Input: part model. Units: mm. Frame: model coordinates. Face numbers are marked on the shaded views. Give positions to 0.01 mm unless a question says otherwise; leave off trailing zeros. Loops run counter-clockwise (first coordinate to the right, second up) from the corner with the lowest first, then second, coordinate; pieces in that order, holes last. Notation, with made-up numbers: (50, 18) -> (61, 18) arc R13 ccw to (61, 27) -> close; hole circle Ø10 at (74.25, 12). An arc over 180 degrees is marked (long way). Answer as a JSON object with one key per item and string values. Group by question number.
```python
from build123d import *

# Parameters (mm, degrees)
SKETCH1_R           = 1.5
SKETCH1_R_2         = 4
BOSS_EXTRUDE1_DEPTH = 3
SKETCH2_R           = 11.5
CUT_EXTRUDE2_DEPTH  = 3
SKETCH3_R           = 5.5
SKETCH3_R_2         = 4
BOSS_EXTRUDE2_DEPTH = 3


with BuildPart() as part:
    # Sketch1 → Boss-Extrude1 (new body)
    with BuildSketch(Plane(origin=(0, 0, 0), x_dir=(1, 0, 0), z_dir=(0, 1, 0))):
        with BuildLine():
            Line((31, -3), (0, -3))
            ThreePointArc((0, -3), (-2.5078369, -1.708002816), (-3.917144015, 0.735837624))
            Line((-3.917144015, 0.735837624), (-7.484880003, 15.5))
            Line((-7.484880003, 15.5), (-2.974611695, 30.760315636))
            ThreePointArc((-2.974611695, 30.760315636), (-1.862648685, 32.724789909), (0, 34))
            Line((0, 34), (31, 34))
            ThreePointArc((31, 34), (34, 31), (31, 28))
            Line((31, 28), (5.467072376, 28))
            Line((5.467072376, 28), (5.467072376, 3))
            Line((5.467072376, 3), (31, 3))
            ThreePointArc((31, 3), (34, 0), (31, -3))
        make_face()
        with Locations((0, 31)):
            Circle(SKETCH1_R, mode=Mode.SUBTRACT)
        with Locations((31, 31)):
            Circle(SKETCH1_R, mode=Mode.SUBTRACT)
        with Locations((31, 0)):
            Circle(SKETCH1_R, mode=Mode.SUBTRACT)
        Circle(SKETCH1_R, mode=Mode.SUBTRACT)
        with Locations((-1.5, 15.5)):
            Circle(SKETCH1_R_2, mode=Mode.SUBTRACT)
    extrude(amount=BOSS_EXTRUDE1_DEPTH)

    # Sketch2 → Cut-Extrude2 (cut)
    with BuildSketch(Plane(origin=(0, 3, 0), x_dir=(1, 0, 0), z_dir=(0, 1, 0))):
        with Locations((15.5, 15.5)):
            Circle(SKETCH2_R)
    extrude(amount=-CUT_EXTRUDE2_DEPTH, mode=Mode.SUBTRACT)

    # Sketch3 → Boss-Extrude2 (add)
    with BuildSketch(Plane(origin=(0, 3, 0), x_dir=(1, 0, 0), z_dir=(0, 1, 0))):
        with Locations((-1.5, 15.5)):
            Circle(SKETCH3_R)
        with Locations((-1.5, 15.5)):
            Circle(SKETCH3_R_2, mode=Mode.SUBTRACT)
    extrude(amount=BOSS_EXTRUDE2_DEPTH)


solid = part.part
```
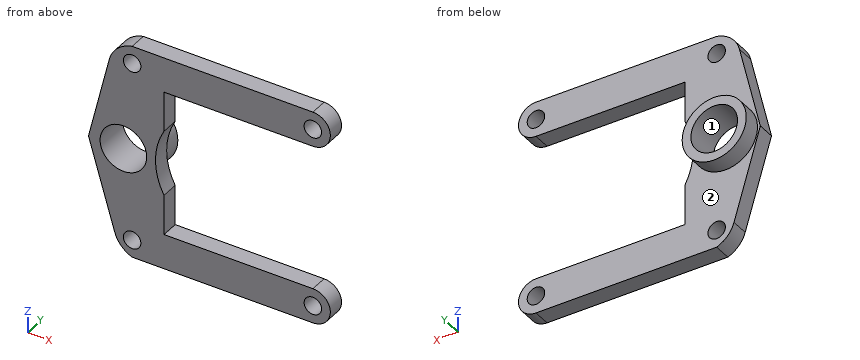
Q1. Section A-A on x = 20. Return the cut outline in (y, z).
Q2. Section B-B on y = 2.35. Return the cut outline in (x, z), then the cut area to 3 significant figures.
Q3. Pin query (flat end, axial travel): pin 1 Ø2.5 at (x, z) = (31, -31) entering from +Y; pin 2 Ø1.5 at (x, y) = (-1.5, 3.5) entering from +Z; pin 3 Ø1.5 at (y, z) = (1.5, -7) entering from +X. Return the tip coordinate at first contact, or that it passes through.
Q4. Ray query, probe 1 along Z at (x, y) = (31, 0.75); probe 2 along X at (y, z) = (1.6, -15.5); probe 3 along Z at (x, y) = (11, 0.35). Return the intervals inside material, ascending.
Q5. Pull-direction query (X, two-part tool) for the marked faces 1 and 2; classes: +X half, -X half, draft (parallel to the pull), parting line (faces both ways), or undercut.
Q6. Section C-C on z = 0. Return the cut outline in (x, y), then the cut area to 3 significant figures.
Q7. Section D-D on z = -18. Return the cut outline in (x, y).
Numbers:
{
 "1": {"outline": "(0, -34) -> (3, -34) -> (3, -28) -> (0, -28) -> close; (0, -3) -> (3, -3) -> (3, 3) -> (0, 3) -> close"},
 "2": {"outline": "(-7.48, -15.5) -> (-2.97, -30.76) arc R5 ccw to (0, -34) -> (31, -34) arc R3 ccw to (31, -28) -> (5.47, -28) -> (5.47, -21.12) arc R11.5 cw to (5.47, -9.88) -> (5.47, -3) -> (31, -3) arc R3 ccw to (31, 3) -> (0, 3) arc R5 ccw to (-3.92, -0.74) -> close; hole circle Ø8 at (-1.5, -15.5); hole circle Ø3 at (0, -31); hole circle Ø3 at (0, 0); hole circle Ø3 at (31, -31); hole circle Ø3 at (31, 0)", "area": "628 mm²"},
 "3": {"pin 1": "passes through", "pin 2": "stops at z = 2.72", "pin 3": "stops at x = 5.47"},
 "4": {"probe 1": "z = -34 to -32.5, -29.5 to -28, -3 to -1.5, 1.5 to 3", "probe 2": "x = -7.48 to -5.5, 2.5 to 4", "probe 3": "z = -34 to -28, -3 to 3"},
 "5": {"face 1": "undercut", "face 2": "draft"},
 "6": {"outline": "(-3.68, 0) -> (-1.5, 0) -> (-1.5, 3) -> (-3.68, 3) -> close; (1.5, 0) -> (29.5, 0) -> (29.5, 3) -> (1.5, 3) -> close; (32.5, 0) -> (34, 0) -> (34, 3) -> (32.5, 3) -> close", "area": "95.0 mm²"},
 "7": {"outline": "(-6.75, 0) -> (-4.62, 0) -> (-4.62, 6) -> (-6.4, 6) -> (-6.4, 3) -> (-6.75, 3) -> close; (1.62, 0) -> (4.28, 0) -> (4.28, 3) -> (3.4, 3) -> (3.4, 6) -> (1.62, 6) -> close"}
}
